Verification items for the finished model (mm, model axes). Face numbers are marked on the shaded views. A direction names the side the tool comes from. Give positions to 0.01 mm unless a question says otherwise; leave off trailing zeros. Write each loop counter-clockwise with the first axis right and the second up, starting at its lowest first coordinate (ties: lowest second). Pieces come first, ordered by that corner, then holes.
Autodesk Fusion 360 part; units mm, degrees
sketch "sketch_for_main_body_shape" plane through (0, 0, 0) normal (0, 0, 1) x (1, 0, 0)
  line L0 (15, -18.5) -> (-15, -18.5) construction
  line L1 (-18.5, -15) -> (-18.5, 15) construction
  line L2 (-15, 18.5) -> (15, 18.5) construction
  line L3 (18.5, 15) -> (18.5, -15) construction
  line L4 (18.5, -18.5) -> (-18.5, 18.5) construction
  line L5 (-18.5, -18.5) -> (18.5, 18.5) construction
  arc A0 (-15, 18.5) -> (-18.5, 15) centre (-15, 15) ccw construction
  arc A1 (-18.5, -15) -> (-15, -18.5) centre (-15, -15) ccw construction
  arc A2 (15, -18.5) -> (18.5, -15) centre (15, -15) ccw construction
  arc A3 (18.5, 15) -> (15, 18.5) centre (15, 15) ccw construction
  arc A4 (19, 15) -> (15, 19) centre (15, 15) ccw
  line L6 (-15, 19) -> (15, 19)
  arc A5 (-15, 19) -> (-19, 15) centre (-15, 15) ccw
  line L7 (-19, -15) -> (-19, 15)
  arc A6 (-19, -15) -> (-15, -19) centre (-15, -15) ccw
  line L8 (15, -19) -> (-15, -19)
  arc A7 (15, -19) -> (19, -15) centre (15, -15) ccw
  line L9 (19, 15) -> (19, -15)
  arc A8 (21.5, 15) -> (15, 21.5) centre (15, 15) ccw
  line L10 (-15, 21.5) -> (15, 21.5)
  arc A9 (-15, 21.5) -> (-21.5, 15) centre (-15, 15) ccw
  line L11 (-21.5, -15) -> (-21.5, 15)
  arc A10 (-21.5, -15) -> (-15, -21.5) centre (-15, -15) ccw
  line L12 (15, -21.5) -> (-15, -21.5)
  arc A11 (15, -21.5) -> (21.5, -15) centre (15, -15) ccw
  line L13 (21.5, 15) -> (21.5, -15)
  circle A12 centre (-15, 15) radius 4
  line L14 (-11, 15) -> (-11, 19)
  line L15 (-15, 11) -> (-19, 11)
  circle A13 centre (15, 15) radius 4
  line L16 (11, 15) -> (11, 19)
  line L17 (15, 11) -> (19, 11)
  line L18 (-37.3211, 0) -> (37.3211, 0) construction
  line L19 (-11, -15) -> (-11, -19)
  circle A14 centre (-15, -15) radius 4
  line L20 (-15, -11) -> (-19, -11)
  circle A15 centre (15, -15) radius 4
  line L21 (15, -11) -> (19, -11)
  line L22 (11, -15) -> (11, -19)
  line L23 (-7.5, -7) -> (-21.5, -7)
  line L24 (-21.5, -7) -> (-21.5, 7)
  line L25 (-21.5, 7) -> (-7.5, 7)
  line L26 (-7.5, 7) -> (-7.5, -7)
  line L27 (21.5, -7) -> (7.5, -7)
  line L28 (7.5, -7) -> (7.5, 7)
  line L29 (7.5, 7) -> (21.5, 7)
  line L30 (21.5, 7) -> (21.5, -7)
  dimension "d6" = 37
  dimension "d7" = 37
  dimension "d8" = 3.5
  dimension "d9" = -0.5
  dimension "d10" = -3
  dimension "d21" = 14
  dimension "d22" = 14
  dimension "d23" = 14
  dimension "d24" = 14
extrude "Extrude1" add sketch "sketch_for_main_body_shape" along normal blind 2
extrude "Extrude2" add sketch "sketch_for_main_body_shape" along normal blind 15 contours A4 L6 A5 L7 L9 A8 L10 A9 L11 L13 A12 A13 L25 L29 | L9 L13 L27 L29 L30 | L7 A6 L8 A7 L9 L11 A10 L12 A11 L13 A14 A15 L23 L27 | L7 L11 L23 L24 L25
extrude "Extrude3" add sketch "sketch_for_main_body_shape" along normal blind 6 contours A4 A13 | L9 A13 L17 | L6 A13 L16 | L6 A12 L14 | A5 A12 | L9 A15 L21 | L7 A12 L15 | A7 A15 | L8 A15 L22 | L8 L19 A14 | L7 A14 L20 | A6 A14
sketch "sketch_for_holes" plane through (0, 0, 6) normal (0, 0, 1) x (-1, 0, 0)
  line L0 (11, -15) -> (11, -19)
  line L1 (11, -19) -> (15, -19)
  arc A0 (15, -19) -> (19, -15) centre (15, -15) ccw
  line L2 (19, -15) -> (19, -11)
  line L3 (19, -11) -> (15, -11)
  arc A1 (15, -11) -> (11, -15) centre (15, -15) ccw
  point P0 (-15, -15)
  point P1 (15, -15)
  point P2 (15, 15)
  point P3 (-15, 15)
hole "Hole1" at (-15, 15, 6) at (15, 15, 6) at (15, -15, 6) at (-15, -15, 6) direction (0, 0, -1) diameter 2.529 depth 4 tip angle 118
extrude "Extrude4" cut sketch "sketch_for_main_body_shape" along normal blind 6 contours L9 L13 L27 L29 L30 | L9 L27 L28 L29 | L7 L23 L25 L26 | L7 L11 L23 L24 L25
sketch "sketch_for_rim" plane through (0, 0, 15) normal (0, 0, 1) x (-1, 0, 0)
  arc A0 (15, -19) -> (19, -15) centre (15, -15) ccw
  line L0 (15, -19) -> (-15, -19)
  arc A1 (-19, -15) -> (-15, -19) centre (-15, -15) ccw
  line L1 (-19, -15) -> (-19, 15)
  arc A2 (-15, 19) -> (-19, 15) centre (-15, 15) ccw
  line L2 (-15, 19) -> (15, 19)
  arc A3 (19, 15) -> (15, 19) centre (15, 15) ccw
  line L3 (19, 15) -> (19, -15)
  arc A4 (15, -21.5) -> (21.5, -15) centre (15, -15) ccw
  line L4 (21.5, -15) -> (21.5, 15)
  arc A5 (21.5, 15) -> (15, 21.5) centre (15, 15) ccw
  line L5 (15, 21.5) -> (-15, 21.5)
  arc A6 (-15, 21.5) -> (-21.5, 15) centre (-15, 15) ccw
  line L6 (-21.5, 15) -> (-21.5, -15)
  arc A7 (-21.5, -15) -> (-15, -21.5) centre (-15, -15) ccw
  line L7 (-15, -21.5) -> (15, -21.5)
  arc A8 (20.5, 15) -> (15, 20.5) centre (15, 15) ccw
  line L8 (-15, 20.5) -> (15, 20.5)
  arc A9 (-15, 20.5) -> (-20.5, 15) centre (-15, 15) ccw
  line L9 (-20.5, -15) -> (-20.5, 15)
  arc A10 (-20.5, -15) -> (-15, -20.5) centre (-15, -15) ccw
  line L10 (15, -20.5) -> (-15, -20.5)
  arc A11 (15, -20.5) -> (20.5, -15) centre (15, -15) ccw
  line L11 (20.5, 15) -> (20.5, -15)
  dimension "d27" = -1.5
extrude "Extrude5" cut sketch "sketch_for_rim" against normal blind 2 contours A8 L8 A9 L9 A10 L10 A11 L11
fillet "Fillet1" radius 3 8 edges at (11, -19, 4) (19, -11, 4) (19, 11, 4) (11, 19, 4) (-11, 19, 4) (-19, 11, 4) (-19, -11, 4) (-11, -19, 4)
fillet "Fillet2" radius 2 4 edges at (7.5, -7, 1) (7.5, 7, 1) (-7.5, 7, 1) (-7.5, -7, 1)
fillet "Fillet3" radius 1.5 4 edges at (-21.5, 7, 3) (-21.5, -7, 3) (21.5, -7, 3) (21.5, 7, 3)
chamfer "Chamfer1" distance 0.5 angle 45 24 edges at (0, -21.5, 0) (-19.5962, -19.5962, 0) (-21.5, -11.75, 0) (-21.0607, -7.4393, 0) (-14.75, -7, 0) (-8.0858, -6.4142, 0) (-7.5, 0, 0) (-8.0858, 6.4142, 0) (-14.75, 7, 0) (-21.0607, 7.4393, 0) (-21.5, 11.75, 0) (-19.5962, 19.5962, 0) (0, 21.5, 0) (19.5962, 19.5962, 0) (21.5, 11.75, 0) (21.0607, 7.4393, 0) (14.75, 7, 0) (8.0858, 6.4142, 0) (7.5, 0, 0) (8.0858, -6.4142, 0) (14.75, -7, 0) (21.0607, -7.4393, 0) (21.5, -11.75, 0) (19.5962, -19.5962, 0)
chamfer "Chamfer2" distance 0.1 angle 45 8 edges at (21.5, 0, 15) (19.5962, 19.5962, 15) (0, 21.5, 15) (-19.5962, 19.5962, 15) (-21.5, 0, 15) (-19.5962, -19.5962, 15) (0, -21.5, 15) (19.5962, -19.5962, 15)
equation "d21 = 11 mm + 3 mm"
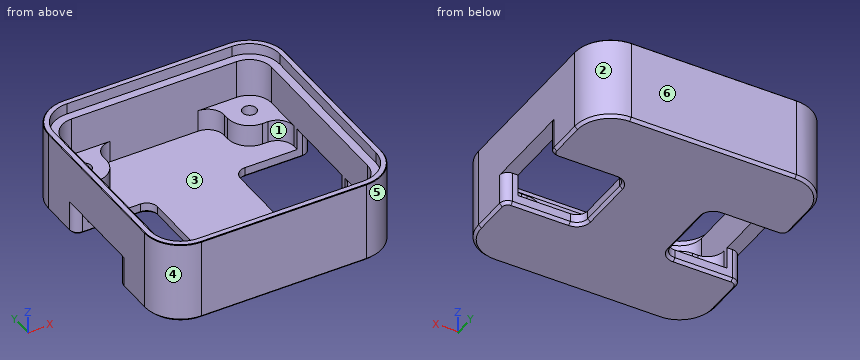
Item 1: Release check for a two-part mould opening along X. For the marked faces 3, 4, 5 and 6 record: released by +X, released by -X, zero draft, split by the parting line, or undercut.
Answer key:
face 3: undercut
face 4: released by -X
face 5: released by +X
face 6: zero draft
Item 2: Depth check by flat-ended pin: pin 1 (0.5 mm diameter, centred on y = 15.5, z = 4, fed in from +X); pin 2 (4 mm diameter, centred on y = -5.5, z = 2.5, fed in from +X); pin 3 (2 mm diameter, centred on x = -6, y = 7.5, fed in from +Z). Enter the tip coordinate at first touch or a pass-through.
Answer key:
pin 1: stops at x = 21.5
pin 2: stops at x = 21.12
pin 3: stops at z = 2
Item 3: Scan lines: line 1 along X through (y, z) = (15, 5.15); line 2 along Y through (x, z) = (9, 14.25). Record each from-to range of solid material in increasing order.
Answer key:
line 1: x = -21.5 to -16.26, -13.74 to -11, 11 to 13.74, 16.26 to 21.5
line 2: y = -21.5 to -20.5, 20.5 to 21.5
Item 4: Set-up check for the marked faces 1 and 2: record each of +Z, -Z, +X, -X, +Y, -Y from which the full face is reachable in a straight line by a thin tool's end or side.
Answer key:
face 1: +Z
face 2: +Z, -Z, +X, +Y
Item 5: Sectioned sample at C-C on x = 0. Record the cut outline in (y, z), then the cut area to 3 significant figures.
Answer key:
outline: (-21.5, 0.5) - (-21, 0) - (21, 0) - (21.5, 0.5) - (21.5, 14.9) - (21.4, 15) - (20.5, 15) - (20.5, 13) - (19, 13) - (19, 2) - (-19, 2) - (-19, 13) - (-20.5, 13) - (-20.5, 15) - (-21.4, 15) - (-21.5, 14.9) - close
area: 145 mm2
Item 6: Sectioned sample at B-B on y = 2.5. Record the cut outline in (x, z).
Answer key:
outline: (-21.5, 6) - (-19, 6) - (-19, 13) - (-20.5, 13) - (-20.5, 15) - (-21.4, 15) - (-21.5, 14.9) - close; (-7.5, 0.5) - (-7, 0) - (7, 0) - (7.5, 0.5) - (7.5, 2) - (-7.5, 2) - close; (19, 6) - (21.5, 6) - (21.5, 14.9) - (21.4, 15) - (20.5, 15) - (20.5, 13) - (19, 13) - close
Item 7: Sectioned sample at A-A on z = 6.75. Record the cut outline in (x, y), then the cut area to 3 significant figures.
Answer key:
outline: (-21.5, -15) arc R6.5 ccw to (-15, -21.5) - (15, -21.5) arc R6.5 ccw to (21.5, -15) - (21.5, 15) arc R6.5 ccw to (15, 21.5) - (-15, 21.5) arc R6.5 ccw to (-21.5, 15) - close; hole (-19, -15) arc R4 ccw to (-15, -19) - (15, -19) arc R4 ccw to (19, -15) - (19, 15) arc R4 ccw to (15, 19) - (-15, 19) arc R4 ccw to (-19, 15) - close
area: 382 mm2
